```python
from build123d import *

# Parameters (mm, degrees)
F1_ANGLE = 180


# Not quite as in the source:
# - a feature names something its author has since deleted; it is built from what else it names


with BuildPart() as f1:
    # F0 (on Right) → F1 (revolve)
    with BuildSketch(Plane.YZ):
        with BuildLine():
            Line((86.8716222048, 33.384835436), (-3.1283777952, 33.384835436))
            Line((-3.1283777952, 33.384835436), (-3.1283777952, 32.384835436))
            Line((-3.1283777952, 32.384835436), (4.0757906815, 32.384835436))
            ThreePointArc((4.0757906815, 32.384835436), (-1.1670524657, 27.9594084914), (-3.1283777952, 21.384835436))
            Line((-3.1283777952, 21.384835436), (-2.1283777952, 21.384835436))
            ThreePointArc((-2.1283777952, 21.384835436), (1.0934476117, 29.1630100291), (8.8716222048, 32.384835436))
            Line((8.8716222048, 32.384835436), (71.8716222048, 32.384835436))
            ThreePointArc((71.8716222048, 32.384835436), (79.3046565784, 29.0966848666), (81.8716222048, 21.384835436))
            Line((81.8716222048, 21.384835436), (83.8716222048, 21.384835436))
            Line((83.8716222048, 21.384835436), (86.8716222048, 23.384835436))
            Line((86.8716222048, 23.384835436), (86.8716222048, 25.384835436))
            Line((86.8716222048, 25.384835436), (85.8716222048, 25.384835436))
            Line((85.8716222048, 25.384835436), (85.8716222048, 23.9200191945))
            Line((85.8716222048, 23.9200191945), (83.568846567, 22.384835436))
            Line((83.568846567, 22.384835436), (82.3074740727, 22.384835436))
            ThreePointArc((82.3074740727, 22.384835436), (80.8426391774, 28.2945551763), (76.3326351779, 32.384835436))
            Line((76.3326351779, 32.384835436), (86.8716222048, 32.384835436))
            Line((86.8716222048, 32.384835436), (86.8716222048, 33.384835436))
        make_face()
    revolve(axis=Axis((0, 40.3716222048, 17.384835436), (0, 1, 0)), revolution_arc=F1_ANGLE)


solid = f1.part
```
The model under review builds one solid part; all positions refer to its coordinate system, in mm. A direction names the side the tool comes from. Round coordinates to 2 decimals unless told otherwise and drop trailing zeros. Order: outer loops, then holes, each group sorted by start corner. A loop starts at its lowest first (then second) coordinate and runs counter-clockwise, first axis right, second up. Notation, with made-up numbers: (-39, 7.5) -> (-19, 7.5) arc R18 ccw to (-19, 41.5) -> close; hole circle Ø5 at (28.25, -12). An arc over 180 degrees is marked (long way). Use a Markdown table: item, result.
Q1. Mouldability with a two-part tool opening along Z and no side actions: class faces 4 (the cylindrical face through (14.996, 0.524, 17.715)), 5 (the flat face through (7, 86.872, 17)), 6 (the cylindrical face through (15.996, 41.242, 17.737)) as +Z half, -Z half, draft (parallel to the pull), parting line (faces both ways), or undercut.
Values:
| item | result |
|---|---|
| face 4 | undercut |
| face 5 | draft |
| face 6 | parting line |
Q2. Tool access review of faces 1 (the cylindrical face through (8, 86.36, 17.56)), 2 (the cylindrical face through (14.996, 40.813, 17.715)), 3 (the conical face through (5.244, 83.937, 17.5)): name each direction out of +Z, -Z, +X, -X, +Y, -Y from which nothing blocks a thin tool from reaching the whole face with its end or side.
Values:
| item | result |
|---|---|
| face 1 | +Y |
| face 2 | -X |
| face 3 | none |
Q3. Clearance check with flat-ended pins moving along their axes: P1, Ø5, axis at x = 8.5, y = 68, coming from the -Z side; P2, Ø6, axis at y = 20, z = 21, coming from the -X side; P3, Ø1, axis at y = 41, z = 27.5, coming from the +X side. State where each tip first meets the part, or that it passes through.
Values:
| item | result |
|---|---|
| P1 | stops at z = 2.55 |
| P2 | stops at x = 13.46 |
| P3 | stops at x = 12.79 |
Q4. We need section A-A on y = 23. Write out the cut boundary in (x, z), then the cut area to 3 significant figures.
Values:
| item | result |
|---|---|
| outline | (0, 1.38) arc R16 ccw to (0, 33.38) -> (0, 32.38) arc R15 cw to (0, 2.38) -> close |
| area | 48.7 mm^2 |
Q5. For line 1 (X direction, y = 71.5, z = 17); line 2 (Y direction, x = 6, z = 23.5); line 3 (Z direction, x = 2.5, y = 42), list the stretches that pass through material, from the lowest coordinate up.
Values:
| item | result |
|---|---|
| line 1 | x = 15 to 16 |
| line 2 | y = -2.23 to -1.14, 81.25 to 81.88 |
| line 3 | z = 1.58 to 2.59, 32.18 to 33.19 |
